CAD build for the part. Positions are in the model's coordinates, mm. Give positions to 0.01 mm unless a question says otherwise; leave off trailing zeros. Write each loop counter-clockwise with the first axis right and the second up, starting at its lowest first coordinate (ties: lowest second). Pieces come first, ordered by that corner, then holes. Notation, with made-up numbers: (-1.5, -7) - (56.5, -7) arc R31 cw to (56.5, 32) - close; hole circle Ø4 at (39.5, 23.5). An arc over 180 degrees is marked (long way). Answer as a JSON object with one key per item and string values.
from build123d import *

# Parameters (mm, degrees)
SKETCH1_R           = 4.25
BASEHEAD_DEPTH      = 5
SKETCH2_R           = 2.5
BASEBODY_DEPTH      = 8
HEXAGONSOCKET_DEPTH = 2.5
TOPFILLET_R         = 0.625
CHAMFER1_SIZE       = 0.2
LPATTERN10_COUNT    = 15
LPATTERN10_PITCH    = 0.5196


with BuildPart() as part:
    # Sketch1 → BaseHead (new body)
    with BuildSketch(Plane(origin=(0, 0, 0), x_dir=(0, 0, -1), z_dir=(1, 0, 0))):
        Circle(SKETCH1_R)
    extrude(amount=BASEHEAD_DEPTH)

    # Sketch2 → BaseBody (add)
    with BuildSketch(Plane(origin=(5, 0, 0), x_dir=(0, 0, -1), z_dir=(1, 0, 0))):
        Circle(SKETCH2_R)
    extrude(amount=BASEBODY_DEPTH)

    # Sketch3 → HexagonSocket (cut)
    with BuildSketch(Plane(origin=(0, 0, 0), x_dir=(0, 0, -1), z_dir=(1, 0, 0))):
        Polygon((2.309401077, 0), (1.154700538, 2), (-1.154700538, 2), (-2.309401077, 0), (-1.154700538, -2), (1.154700538, -2), align=None)
    extrude(amount=HEXAGONSOCKET_DEPTH, mode=Mode.SUBTRACT)

    # Sketch4 → Cut-Revolve1 (revolve, cut)
    with BuildSketch(Plane(origin=(-4.19613823, 0.75, 0), x_dir=(-1, 0, 0), z_dir=(0, 0, 1))):
        Polygon((-6.69613823, 2.75), (-7.850838768, 0.75), (-6.69613823, 0.75), align=None)
    revolve(axis=Axis((0.838992387, 0, 0), (-1, 0, 0)), mode=Mode.SUBTRACT)

    # TopFillet
    topfillet_edges = [part.edges().sort_by_distance(p)[0] for p in [
        (0, 0, 4.25),
    ]]
    fillet(topfillet_edges, radius=TOPFILLET_R)

    # Chamfer1
    chamfer1_edges = [part.edges().sort_by_distance(p)[0] for p in [
        (13, 0, 2.5),
    ]]
    chamfer(chamfer1_edges, length=CHAMFER1_SIZE)

    # Sketch5 → Cut-Revolve10 (revolve, cut)
    with BuildSketch(Plane.XY):
        Polygon((12.8, 2.125011), (13.0165, 2.5), (13.0165, 2.933), (12.5835, 2.933), (12.5835, 2.5), align=None)
    cut_revolve10 = revolve(axis=Axis((0, 0, 0), (1, 0, 0)), mode=Mode.SUBTRACT)

    # LPattern10: Cut-Revolve10 ×15
    with Locations(*[(-i * LPATTERN10_PITCH, 0, 0) for i in range(1, LPATTERN10_COUNT)]):
        add(cut_revolve10, mode=Mode.SUBTRACT)


solid = part.part
Item 1: Mould opens along Y. For faces 1 (the flat face through (1, -2, 0)), 2 (the flat face through (1.23, 0.99, -1.74)), 3 (the flat face through (5, -2, -2)) say: +Y half, -Y half, draft (parallel to the pull), parting line (faces both ways), or undercut.
Entries:
{"face 1": "undercut", "face 2": "undercut", "face 3": "draft"}
Item 2: Probe line 1 (Y direction, x = 2.75, z = -3.75); line 2 (X direction, y = 0.5, z = 3); line 3 (Z direction, x = 1.5, y = 0.5). List the from-to ranges inside material, lowest first. Write a range as from..to.
Entries:
{"line 1": "-2..2", "line 2": "0..5", "line 3": "-4.22..-2.02, 2.02..4.22"}
Item 3: Flat gauge pins, fed straight in: P1, Ø3, axis at x = 11, z = -2, coming from the -Y side; P2, Ø1.5, axis at x = 11, y = -3, coming from the +Z side; P3, Ø1.5, axis at x = 8.5, z = -3, coming from the +Y side. Where does each tip first touch, or does it go through?
Entries:
{"P1": "y = -2.45", "P2": "z = 1.09", "P3": "y = 1.08"}
Item 4: Cut at A-A (x = 3.25). Give the cut face in (y, z).
Entries:
{"outline": "circle Ø8.5 at (0, 0); hole circle Ø1.4 at (0, 0)"}
